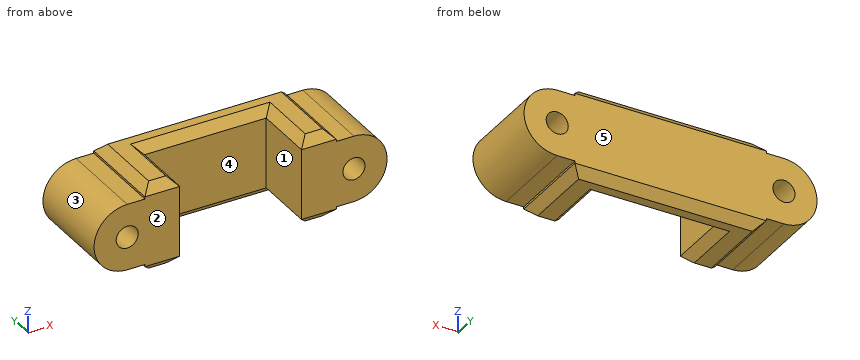
```python
from build123d import *

# Parameters (mm, degrees)
F1_DEPTH = 25.4
F2_R     = 3.175
F3_DEPTH = 25.4
F4_SIZE  = 2.54


with BuildPart() as f1:
    # F0 (on Top) → F1 (new body)
    with BuildSketch(Plane.XY):
        Polygon((-17.5, 17.5), (17.5, 17.5), (17.5, 0), (27.5, 0), (27.5, 25.4), (-27.5, 25.4), (-27.5, 0), (-17.5, 0), align=None)
    extrude(amount=F1_DEPTH)

    # F2 (on Front) → F3 (join)
    with BuildSketch(Plane.XZ):
        with BuildLine():
            Line((-27.5, 3.175), (-27.5, 22.225))
            Line((-27.5, 22.225), (-32.58, 22.225))
            ThreePointArc((-32.58, 22.225), (-42.105, 12.7), (-32.58, 3.175))
            Line((-32.58, 3.175), (-27.5, 3.175))
        make_face()
        with Locations((-32.58, 12.7)):
            Circle(F2_R, mode=Mode.SUBTRACT)
    extrude(amount=-F3_DEPTH)

    # F4
    f4_edges = [f1.edges().sort_by_distance(p)[0] for p in [
        (0, 17.5, 0),
        (17.5, 8.75, 0),
        (22.5, 0, 0),
        (27.5, 12.7, 0),
        (0, 25.4, 0),
        (-27.5, 12.7, 0),
        (-22.5, 0, 0),
        (-17.5, 8.75, 0),
        (0, 17.5, 25.4),
        (17.5, 8.75, 25.4),
        (22.5, 0, 25.4),
        (27.5, 12.7, 25.4),
        (0, 25.4, 25.4),
        (-27.5, 12.7, 25.4),
        (-22.5, 0, 25.4),
        (-17.5, 8.75, 25.4),
    ]]
    chamfer(f4_edges, length=F4_SIZE)

    # F5: F1 across plane


with BuildPart() as f1_1:
    add(f1.part)
    add(f1.part.mirror(Plane.YZ))


solid = f1_1.part
```
Check sheet for the modelled part. Datum: model origin and axes. Units: mm. Face numbers are marked on the shaded views. A direction names the side the tool comes from. Round coordinates to 2 decimals unless told otherwise and drop trailing zeros. Loops run counter-clockwise (first coordinate to the right, second up) from the corner with the lowest first, then second, coordinate; pieces in that order, holes last. Notation, with made-up numbers: M -21.5,-18.5 L -5.5,-18.5 A18 ccw -5.5,-7.5 Z; hole C 87,68 d6. An arc over 180 degrees is marked long. Answer as a JSON object with one key per item and string values.
1. Section check A-A (z = 12.7). Record the boundary of the cut face in (x, y) (3 decimals).
Reply:
{"outline": "M -42.105,0 L -35.755,0 L -35.755,25.4 L -42.105,25.4 Z; M -29.405,0 L -17.5,0 L -17.5,17.5 L 17.5,17.5 L 17.5,0 L 29.405,0 L 29.405,25.4 L -29.405,25.4 Z; M 35.755,0 L 42.105,0 L 42.105,25.4 L 35.755,25.4 Z"}
2. Access from +Z, -Z, +X, -X, +Y, -Y to the whole of each face (thin tool, end or side, straight path). Record for the marked faces 4 and 5.
Reply:
{"face 4": "+Z, -Z, -Y", "face 5": "+Z, -Z, +X, -X, +Y"}
3. Mould release check, pull along X, two halves, no side actions. Record for the marked faces 1, 2 and 3: pulls with the +X half, pulls with the -X half, needs draft (parallel to the pull), parting line crosses it, or undercut.
Reply:
{"face 1": "undercut", "face 2": "needs draft", "face 3": "pulls with the -X half"}
4. Section check B-B (y = 18.5). Record the boundary of the cut face in (x, z) (3 decimals).
Reply:
{"outline": "M -32.58,3.175 L -27.5,3.175 L -27.5,2.54 L -24.96,0 L -20.04,0 L -18.5,1.54 L 18.5,1.54 L 20.04,0 L 24.96,0 L 27.5,2.54 L 27.5,3.175 L 32.58,3.175 A9.525 ccw 32.58,22.225 L 27.5,22.225 L 27.5,22.86 L 24.96,25.4 L 20.04,25.4 L 18.5,23.86 L -18.5,23.86 L -20.04,25.4 L -24.96,25.4 L -27.5,22.86 L -27.5,22.225 L -32.58,22.225 A9.525 ccw Z; hole C -32.58,12.7 d6.35; hole C 32.58,12.7 d6.35"}
5. Gauge pin test, flat ends, axial feed: P1, Ø10, axis at y = 17.5, z = 13, coming from the -X side (3 decimals); P2, Ø10, axis at x = 0, z = 12.5, coming from the -Y side; P3, Ø5.5, axis at x = -29, y = 8, coming from the -Z side; P4, Ø5.5, axis at x = 31, y = 14, coming from the -Z side (3 decimals). Record the tip position at first contact, or that the pin passes through.
Reply:
{"P1": "stops at x = -42.105", "P2": "stops at y = 17.5", "P3": "stops at z = 1.29", "P4": "stops at z = 3.175"}
6. Scan lines: line 1 (Z direction, x = 32.58, y = 17.25) (3 decimals); line 2 (X direction, y = 8, z = 5.75); line 3 (X direction, y = 12, z = 6.5). Record each from-to range of solid material in increasing order.
Reply:
{"line 1": "z = 3.175 to 9.525, 15.875 to 22.225", "line 2": "x = -39.09 to -17.5, 17.5 to 39.09", "line 3": "x = -39.81 to -17.5, 17.5 to 39.81"}
7. Section check C-C (y = 6.5). Record the boundary of the cut face in (x, z) (3 decimals).
Reply:
{"outline": "M -32.58,3.175 L -27.5,3.175 L -27.5,2.54 L -24.96,0 L -20.04,0 L -17.5,2.54 L -17.5,22.86 L -20.04,25.4 L -24.96,25.4 L -27.5,22.86 L -27.5,22.225 L -32.58,22.225 A9.525 ccw Z; M 17.5,2.54 L 20.04,0 L 24.96,0 L 27.5,2.54 L 27.5,3.175 L 32.58,3.175 A9.525 ccw 32.58,22.225 L 27.5,22.225 L 27.5,22.86 L 24.96,25.4 L 20.04,25.4 L 17.5,22.86 Z; hole C -32.58,12.7 d6.35; hole C 32.58,12.7 d6.35"}
8. Section check D-D (x = 34). Record the boundary of the cut face in (y, z).
Reply:
{"outline": "M 0,3.28 L 25.4,3.28 L 25.4,9.86 L 0,9.86 Z; M 0,15.54 L 25.4,15.54 L 25.4,22.12 L 0,22.12 Z"}
